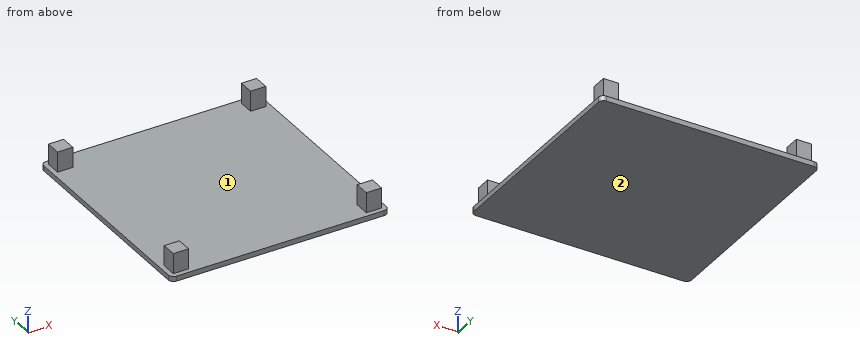
```python
from build123d import *

# Parameters (mm, degrees)
SKETCH_W     = 43
SKETCH_H     = 43
PAD_DEPTH    = 1
SKETCH001_W  = 3
SKETCH001_H  = 3
PAD001_DEPTH = 4
FILLET_R     = 1
FILLET001_R  = 1
FILLET002_R  = 1
FILLET003_R  = 1


with BuildPart() as part:
    # Sketch → Pad (new body)
    with BuildSketch(Plane.XY):
        Rectangle(SKETCH_W, SKETCH_H)
    extrude(amount=PAD_DEPTH)

    # Sketch001 (on Face6 of Pad) → Pad001 (join)
    with BuildSketch(Plane.XY.offset(1)):
        with Locations((-19.05, 19.05)):
            Rectangle(SKETCH001_W, SKETCH001_H)
        with Locations((19.05, 19.05)):
            Rectangle(SKETCH001_W, SKETCH001_H)
        with Locations((-19.05, -19.05)):
            Rectangle(SKETCH001_W, SKETCH001_H)
        with Locations((19.05, -19.05)):
            Rectangle(SKETCH001_W, SKETCH001_H)
    extrude(amount=PAD001_DEPTH)

    # Fillet
    fillet_edges = [part.edges().sort_by_distance(p)[0] for p in [
        (-21.5, -21.5, 0.5),
    ]]
    fillet(fillet_edges, radius=FILLET_R)

    # Fillet001
    fillet001_edges = [part.edges().sort_by_distance(p)[0] for p in [
        (21.5, -21.5, 0.5),
    ]]
    fillet(fillet001_edges, radius=FILLET001_R)

    # Fillet002
    fillet002_edges = [part.edges().sort_by_distance(p)[0] for p in [
        (-21.5, 21.5, 0.5),
    ]]
    fillet(fillet002_edges, radius=FILLET002_R)

    # Fillet003
    fillet003_edges = [part.edges().sort_by_distance(p)[0] for p in [
        (21.5, 21.5, 0.5),
    ]]
    fillet(fillet003_edges, radius=FILLET003_R)


solid = part.part
```
For this review, take the finished solid that the model builds, in its own axes (mm). Face numbers are marked on the shaded views. Round coordinates to 2 decimals unless told otherwise and drop trailing zeros. Write each loop counter-clockwise with the first axis right and the second up, starting at its lowest first coordinate (ties: lowest second). Pieces come first, ordered by that corner, then holes. Notation, with made-up numbers: (18.5, 85.5) - (61.5, 85.5) arc R17 cw to (61.5, 115.5) - close; hole circle Ø5 at (-11, 77.25). An arc over 180 degrees is marked (long way). Use CSV: the item, a comma, the result in double quotes.
1) Add section A-A on z = 2.7. Write out the cut boundary in (x, y), and give its area (3 significant figures).
Conclusion:
outline,"(-20.55, -20.55) - (-17.55, -20.55) - (-17.55, -17.55) - (-20.55, -17.55) - close; (-20.55, 17.55) - (-17.55, 17.55) - (-17.55, 20.55) - (-20.55, 20.55) - close; (17.55, -20.55) - (20.55, -20.55) - (20.55, -17.55) - (17.55, -17.55) - close; (17.55, 17.55) - (20.55, 17.55) - (20.55, 20.55) - (17.55, 20.55) - close"
area,"36.0 mm^2"
2) The part is to be moulded in two halves that separate along Y. For the marked faces 1 and 2, say which applies: pulls with the +Y half, pulls with the -Y half, needs draft (parallel to the pull), parting line crosses it, or undercut.
Conclusion:
face 1,"undercut"
face 2,"needs draft"
3) Clearance check with flat-ended pins moving along their axes: pin 1 Ø2.5 at (y, z) = (19, 2.5) entering from -X; pin 2 Ø1.5 at (x, z) = (20, 3) entering from +Y; pin 3 Ø2 at (x, y) = (10.5, 5.5) entering from +Z. State where each tip first meets the part, or that it passes through.
Conclusion:
pin 1,"stops at x = -20.55"
pin 2,"stops at y = 20.55"
pin 3,"stops at z = 1"
4) Add section B-B on x = 4.5. Write out the cut boundary in (y, z).
Conclusion:
outline,"(-21.5, 0) - (21.5, 0) - (21.5, 1) - (-21.5, 1) - close"
5) Wall thickness on line 1 along X through (y, z) = (19.5, 4.1); line 2 along Z through (x, y) = (7, -15): over which ranges is each line inside the solid? List them lowest first. Write a range as from..to.
Conclusion:
line 1,"x = -20.55..-17.55, 17.55..20.55"
line 2,"z = 0..1"
